Can you work these out from the model? Positions are in its coordinate system, mm. Face numbers are marked on the shaded views. A direction names the side the tool comes from. Coordinates: 2 decimals unless noted, no trailing zeros. Order: outer loops, then holes, each group sorted by start corner. A loop starts at its lowest first (then second) coordinate and runs counter-clockwise, first axis right, second up. Notation, with made-up numbers: (81.5, 40) - (100.5, 40) arc R8 ccw to (100.5, 52) - close; hole circle Ø1 at (54.5, 10.5). An arc over 180 degrees is marked (long way). Use a Markdown table: item, result. Add a question column.
(1) On a 3-axis mill with a long thin cutter (end or side, diameter ignored), from which of +Z, -Z, +X, -X, +Y, -Y can I reach the whole of each face in a straight line? I mean the marked faces 4, 5, 6 and 7. Say none if no direction works.
(2) I want a section at B-B (z = 11). List the corners of the cut face in (x, y) for me.
(3) I want a section at A-A (x = 6.5). List the corners of the cut face in (y, z) for me.
(4) I want a section at D-D (y = 2.75). List the corners of the cut face in (x, z) for me.
(5) I want a section at C-C (y = 10). List the corners of the cut face in (x, z) for me.
(6) For pin 1 Ø2.5 at (y, z) = (13.5, 44) entering from +X; pin 2 Ø5.5 at (y, z) = (23, 46.5) entering from +X; pin 3 Ø15 at (y, z) = (5, 11) entering from +X; pin 4 Ø6.5 at (x, y) = (34, 10) entering from -Z, each with a flat end and sliding along its axis, tell me the tip position at first contact or that it passes through.
(7) If I drill on L1, parallel to X at y = 9.75, z = 44; L2, parallel to Y at x = 34, z = -27.5; L3, parallel to Z at x = -3, y = 13, over which ranges is the centre line in solid material (lowest first)? Write a range as [from, to].
(8) We'd pull the mould along X, two halves only. Please class the marked faces 1, 2 and 3: pulls with the +X half, pulls with the -X half, needs draft (parallel to the pull), parting line crosses it, or undercut.
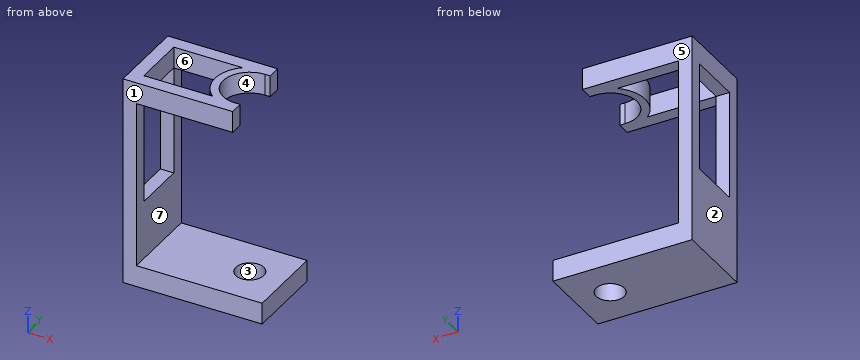
```python
from build123d import *

# Parameters (mm, degrees)
SKETCH011_W     = 30
SKETCH011_H     = 78.5
SKETCH011_W_2   = 20
SKETCH011_H_2   = 40.5
PAD009_DEPTH    = 5
SKETCH008_W     = 30
SKETCH008_H     = 8
PAD008_DEPTH    = 47
SKETCH009_W     = 5
SKETCH009_H     = 8
PAD012_DEPTH    = 36
PAD010_DEPTH    = 8
SKETCH012_R     = 1.5
POCKET004_DEPTH = 6.501
SKETCH015_R     = 5.25
POCKET003_DEPTH = 30.001


with BuildPart() as part:
    # Sketch011 → Pad009 (new body)
    with BuildSketch(Plane.YZ):
        with Locations((10, 9.25)):
            Rectangle(SKETCH011_W, SKETCH011_H)
        with Locations((10, 20.25)):
            Rectangle(SKETCH011_W_2, SKETCH011_H_2, mode=Mode.SUBTRACT)
    extrude(amount=-PAD009_DEPTH)

    # Sketch008 → Pad008 (join)
    with BuildSketch(Plane.YZ):
        with Locations((10, -26)):
            Rectangle(SKETCH008_W, SKETCH008_H)
    extrude(amount=PAD008_DEPTH)

    # Sketch009 → Pad012 (join)
    with BuildSketch(Plane.YZ):
        with Locations((-2.5, 44.5)):
            Rectangle(SKETCH009_W, SKETCH009_H)
        with Locations((22.5, 44.5)):
            Rectangle(SKETCH009_W, SKETCH009_H)
    extrude(amount=PAD012_DEPTH)

    # Sketch010 → Pad010 (join)
    with BuildSketch(Plane.XY.offset(40.5)):
        with BuildLine():
            ThreePointArc((34, 20), (24, 10), (34, 0))
            Line((34, 0), (34, -5))
            Line((34, -5), (31, -5))
            Line((31, -5), (31, -2.649111))
            ThreePointArc((31, 22.649111), (21, 10), (31, -2.649111))
            Line((31, 25), (31, 22.649111))
            Line((34, 25), (31, 25))
            Line((34, 20), (34, 25))
        make_face()
    extrude(amount=PAD010_DEPTH)

    # Sketch012 → Pocket004 (cut, through all)
    with BuildSketch(Plane.YZ.offset(40.5)):
        with Locations((-2.5, 44.5)):
            Circle(SKETCH012_R)
        with Locations((22.5, 44.5)):
            Circle(SKETCH012_R)
    extrude(amount=POCKET004_DEPTH, mode=Mode.SUBTRACT)

    # Sketch015 → Pocket003 (cut, through all)
    with BuildSketch(Plane.XY):
        with Locations((34, 10)):
            Circle(SKETCH015_R)
    extrude(amount=-POCKET003_DEPTH, mode=Mode.SUBTRACT)


solid = part.part
```
Answers follow:
| question | item | result |
|---|---|---|
| 1 | face 4 | +Z, +X |
| 1 | face 5 | +Z, -Z, +X, -X, +Y |
| 1 | face 6 | +Z |
| 1 | face 7 | +X, +Y, -Y |
| 2 | outline | (-5, -5) - (0, -5) - (0, 0) - (-5, 0) - close; (-5, 20) - (0, 20) - (0, 25) - (-5, 25) - close |
| 3 | outline | (-5, -30) - (25, -30) - (25, -22) - (-5, -22) - close; (-5, 40.5) - (0, 40.5) - (0, 48.5) - (-5, 48.5) - close; (20, 40.5) - (25, 40.5) - (25, 48.5) - (20, 48.5) - close |
| 4 | outline | (-5, -30) - (47, -30) - (47, -22) - (0, -22) - (0, 0) - (-5, 0) - close; (-5, 40.5) - (0, 40.5) - (0, 48.5) - (-5, 48.5) - close; (23.21, 40.5) - (27.11, 40.5) - (27.11, 48.5) - (23.21, 48.5) - close |
| 5 | outline | (-5, -30) - (28.75, -30) - (28.75, -22) - (0, -22) - (0, 0) - (-5, 0) - close; (-5, 40.5) - (0, 40.5) - (0, 48.5) - (-5, 48.5) - close; (21, 40.5) - (24, 40.5) - (24, 48.5) - (21, 48.5) - close; (39.25, -30) - (47, -30) - (47, -22) - (39.25, -22) - close |
| 6 | pin 1 | stops at x = 25.2 |
| 6 | pin 2 | stops at x = 36 |
| 6 | pin 3 | stops at x = 0 |
| 6 | pin 4 | passes through |
| 7 | L1 | x = [-5, 0], [21, 24] |
| 7 | L2 | y = [-5, 4.75], [15.25, 25] |
| 7 | L3 | z = [-30, 0], [40.5, 48.5] |
| 8 | face 1 | needs draft |
| 8 | face 2 | pulls with the -X half |
| 8 | face 3 | undercut |
